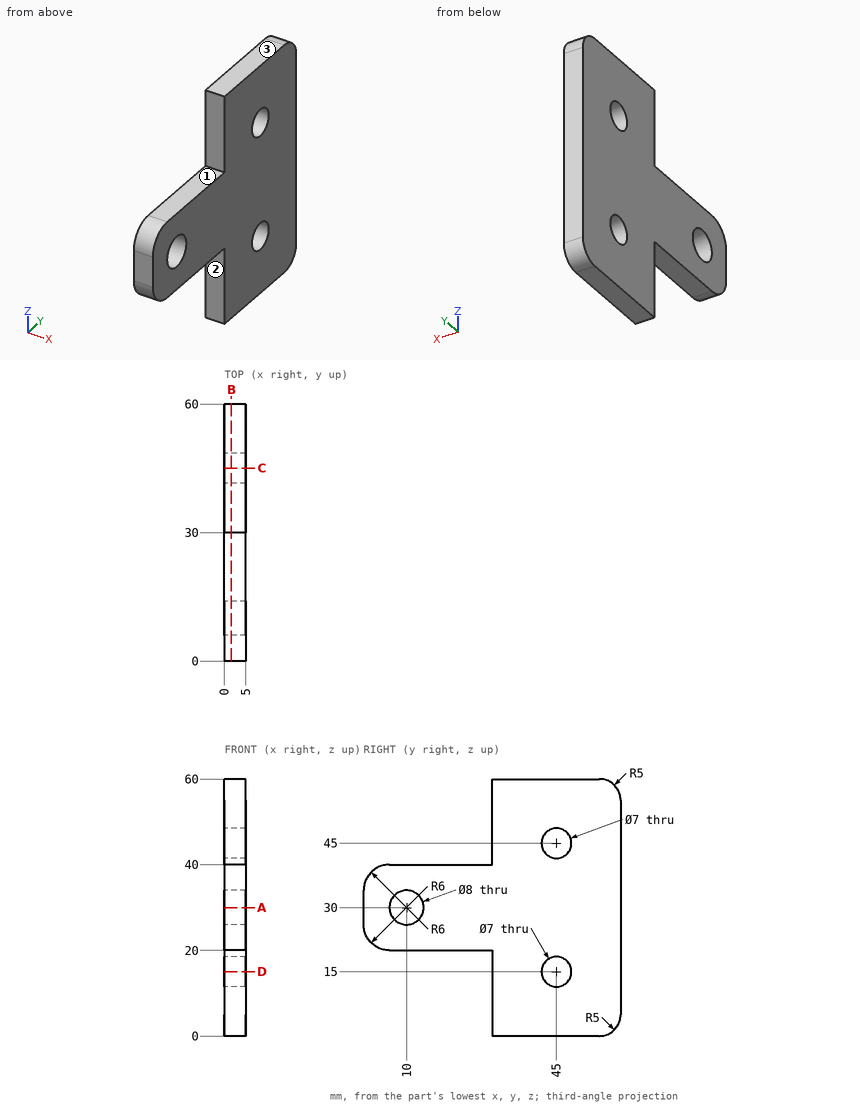
Could you check a few things on this drawing? It's one solid part, dimensions in mm from its lowest x, y, z. A direction names the side the tool comes from. Round coordinates to 2 decimals unless told otherwise and drop trailing zeros. Write each loop counter-clockwise with the first axis right and the second up, starting at its lowest first coordinate (ties: lowest second). Pieces come first, ordered by that corner, then holes. Notation, with made-up numbers: M 56,60.5 L 110,60.5 A20 cw 110,91.5 Z; hole C 15.5,-23.75 d4. An arc over 180 degrees is marked long. Answer as CSV lines item,"result". Start each with the question number.
1. I need wall thicknesses on probe 1 along Z at (x, y) = (3.75, 45); probe 2 along Z at (x, y) = (3.25, 10); probe 3 along Z at (x, y) = (2.75, 19). Which ranges of each line are inside material? Lowest first, please.
2. Suppose I cut it at C-C on y = 45. Write out the boundary of the cut face in (x, z), then the cut area to 3 significant figures.
3. I'm going to push flat-ended pins straight in: pin 1 Ø1 at (x, y) = (3.5, 23) entering from +Z; pin 2 Ø2.5 at (x, y) = (3.5, 23) entering from -Z. Where does each tip first touch, or does it pass through?
4. Suppose I cut it at A-A on z = 30. Write out the boundary of the cut face in (x, y), then the cut area to 3 significant figures.
5. Suppose I cut it at D-D on z = 15. Write out the boundary of the cut face in (x, y).
6. Suppose I cut it at B-B on x = 1.65. Write out the boundary of the cut face in (y, z), then the cut area to 3 significant figures.
7. On a 3-axis mill with a long thin cutter (end or side, diameter ignored), from which of +Z, -Z, +X, -X, +Y, -Y can I reach the whole of each face in a straight line? I mean the marked faces 1, 2 and 3. Say none if no direction works.
Check result:
1,probe 1,"z = 0 to 11.5, 18.5 to 41.5, 48.5 to 60"
1,probe 2,"z = 20 to 26, 34 to 40"
1,probe 3,"z = 20 to 40"
2,outline,"M 0,0 L 5,0 L 5,11.5 L 0,11.5 Z; M 0,18.5 L 5,18.5 L 5,41.5 L 0,41.5 Z; M 0,48.5 L 5,48.5 L 5,60 L 0,60 Z"
2,area,"230 mm2"
3,pin 1,"stops at z = 40"
3,pin 2,"stops at z = 20"
4,outline,"M 0,0 L 5,0 L 5,6 L 0,6 Z; M 0,14 L 5,14 L 5,60 L 0,60 Z"
4,area,"260 mm2"
5,outline,"M 0,30 L 5,30 L 5,41.5 L 0,41.5 Z; M 0,48.5 L 5,48.5 L 5,60 L 0,60 Z"
6,outline,"M 0,26 A6 ccw 6,20 L 30,20 L 30,0 L 55,0 A5 ccw 60,5 L 60,55 A5 ccw 55,60 L 30,60 L 30,40 L 6,40 A6 ccw 0,34 Z; hole C 10,30 d8; hole C 45,15 d7; hole C 45,45 d7"
6,area,"2,250 mm2"
7,face 1,"+Z, +X, -X, -Y"
7,face 2,"-Z, +X, -X, -Y"
7,face 3,"+Z, +X, -X, +Y, -Y"
